Answer from the drawing. Dimensions are ordinates in mm from the lowest x, y and z of the part. A direction names the side the tool comes from. Round coordinates to 2 decimals unless told otherwise and drop trailing zeros. Loops run counter-clockwise (first coordinate to the right, second up) from the corner with the lowest first, then second, coordinate; pieces in that order, holes last.
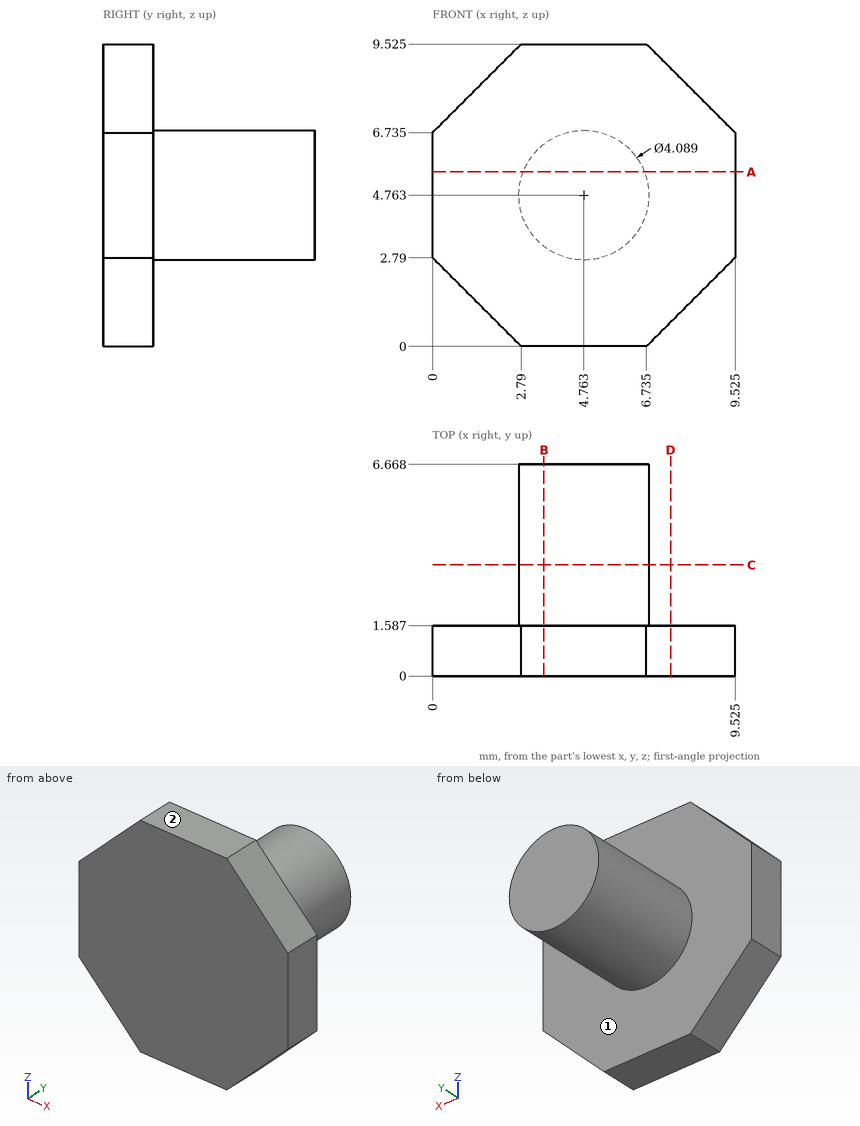
1. Given pin 1 (1.5 mm diameter, centred on x = 5, z = 1.5, fed in from +Y), flat-ended and moving along its own axis, determine where the tip first touches the part or whether it passes through.
Answer key:
pin 1: stops at y = 1.59
2. Find section A-A (z = 5.5). Write down the section's boundary in (x, y) (1 decimal), then the cut area to 3 significant figures.
Answer key:
outline: (0, 0) - (9.5, 0) - (9.5, 1.6) - (6.7, 1.6) - (6.7, 6.7) - (2.9, 6.7) - (2.9, 1.6) - (0, 1.6) - close
area: 34.5 mm2
3. Consider probe 1 along Y at (x, z) = (7.5, 6); probe 2 along Z at (x, y) = (4, 4) (1 decimal); probe 3 along X at (y, z) = (3.75, 3.75) (1 decimal). Determine where each line is inside the solid, lowest interval first.
Answer key:
probe 1: y = 0 to 1.59
probe 2: z = 2.9 to 6.7
probe 3: x = 3 to 6.5
4. Find section C-C (y = 3.5). Write down the section's boundary in (x, z) (1 decimal).
Answer key:
outline: circle Ø4.1 at (4.8, 4.8)
5. Find section D-D (x = 7.5). Write down the section's boundary in (y, z) (1 decimal), then the cut area to 3 significant figures.
Answer key:
outline: (0, 0.8) - (1.6, 0.8) - (1.6, 8.8) - (0, 8.8) - close
area: 12.7 mm2
6. Which of the six approach directions +Z, -Z, +X, -X, +Y, -Y give full straight-line access (tool end or side, diameter ignored) to the marked faces 1 and 2?
Answer key:
face 1: +Y
face 2: +Z, +X, -X, +Y, -Y
7. Find section B-B (x = 3.5). Write down the section's boundary in (y, z) (1 decimal).
Answer key:
outline: (0, 0) - (1.6, 0) - (1.6, 3.2) - (6.7, 3.2) - (6.7, 6.4) - (1.6, 6.4) - (1.6, 9.5) - (0, 9.5) - close
